```python
from build123d import *

# Parameters (mm, degrees)
SKETCH2_R          = 2.5
CUT_EXTRUDE1_DEPTH = 7


with BuildPart() as part:
    # Sketch1 → Revolve1 (revolve)
    with BuildSketch(Plane.XY):
        Polygon((0, 16), (0, 34), (-6, 34), (-6, 22), (-18, 22), (-18, 10.5), (-12, 10.5), (-12, 16), align=None)
    revolve(axis=Axis((-41.962696156, 0, 0), (1, 0, 0)))

    # Sketch2 → Cut-Extrude1 (cut, through all)
    with BuildSketch(Plane.ZY.offset(6)):
        with Locations((0, 28)):
            Circle(SKETCH2_R)
        with Locations((28, 0)):
            Circle(SKETCH2_R)
        with Locations((0, -28)):
            Circle(SKETCH2_R)
        with Locations((-28, 0)):
            Circle(SKETCH2_R)
    extrude(amount=-CUT_EXTRUDE1_DEPTH, mode=Mode.SUBTRACT)


solid = part.part
```
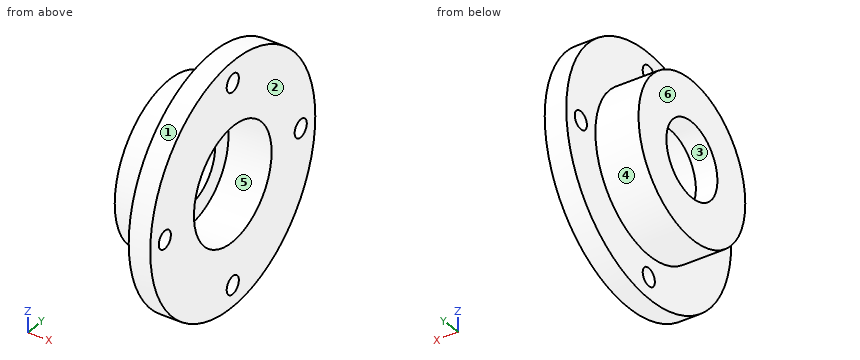
The model under review builds one solid part; all positions refer to its coordinate system, in mm. Face numbers are marked on the shaded views. A direction names the side the tool comes from. Give positions to 0.01 mm unless a question says otherwise; leave off trailing zeros. Order: outer loops, then holes, each group sorted by start corner. A loop starts at its lowest first (then second) coordinate and runs counter-clockwise, first axis right, second up. Notation, with made-up numbers: (-28.75, -17.5) - (-21.75, -17.5) arc R14 cw to (-21.75, 1.5) - close; hole circle Ø5 at (0.5, 50). An arc over 180 degrees is marked (long way). Use CSV: the item, a comma, the result in double quotes. Start each with the question number.
Q1. We need section B-B, the plane x = -15.25. Write out the cut boundary in (y, z), and give its area (3 significant figures).
Q2. We need section D-D, the plane y = -13. Write out the cut boundary in (x, z).
Q3. Tool access review of the marked faces 4, 5 and 6: name each direction out of +Z, -Z, +X, -X, +Y, -Y from which nothing blocks a thin tool from reaching the whole face with its end or side.
Q4. To check wall thickness, follow line 1 along Z through (x, y) = (-14.2, 0); line 2 along X through (y, z) = (-4, -11); line 3 along Z through (x, y) = (-2.5, -30). State the ranges of each line that lie inside material, in increasing order. Write a range as [from, to].
Q5. Clearance check with flat-ended pins moving along their axes: pin 1 Ø6 at (x, z) = (-5.5, -11.5) entering from -Y; pin 2 Ø1.5 at (x, z) = (-12.5, -6.5) entering from +Y; pin 3 Ø3 at (x, z) = (-10, 19) entering from +Y. State where each tip first meets the part, or that it passes through.
Q6. The part is to be moulded in two halves that separate along Y. For the marked faces 1, 2 and 3, say which applies: +Y half, -Y half, draft (parallel to the pull), parting line (faces both ways), or undercut.
Q7. We need section A-A, the plane y = -28. Write out the cut boundary in (x, z), and give its area (3 significant figures).
Outcome:
1,outline,"circle Ø44 at (0, 0); hole circle Ø21 at (0, 0)"
1,area,"1,170 mm^2"
2,outline,"(-18, -17.75) - (-6, -17.75) - (-6, -31.42) - (0, -31.42) - (0, -9.33) - (-12, -9.33) - (-12, 9.33) - (0, 9.33) - (0, 31.42) - (-6, 31.42) - (-6, 17.75) - (-18, 17.75) - close"
3,face 4,"-X"
3,face 5,"+X"
3,face 6,"+Z, -Z, -X, +Y, -Y"
4,line 1,"z = [-22, -10.5], [10.5, 22]"
4,line 2,"x = [-18, -12]"
4,line 3,"z = [-16, -1.5], [1.5, 16]"
5,pin 1,"stops at y = -32.92"
5,pin 2,"stops at y = 21.24"
5,pin 3,"stops at y = 13.33"
6,face 1,"parting line"
6,face 2,"draft"
6,face 3,"undercut"
7,outline,"(-6, -19.29) - (0, -19.29) - (0, -2.5) - (-6, -2.5) - close; (-6, 2.5) - (0, 2.5) - (0, 19.29) - (-6, 19.29) - close"
7,area,"201 mm^2"
